Autodesk Inventor part; units mm, degrees
ref_plane "YZ Plane" through (0, 0, 0) normal (1, 0, 0) x (0, 1, 0)
ref_plane "XZ Plane" through (0, 0, 0) normal (0, 1, 0) x (-1, 0, 0)
ref_plane "XY Plane" through (0, 0, 0) normal (0, 0, 1) x (1, 0, 0)
sketch "Sketch1" plane through (0, 0, 0) normal (0, 1, 0) x (-1, 0, 0)
  line L0 (0, 0) -> (15.5956, 0)
  line L1 (15.5956, 0) -> (15.5956, -46.7868)
  line L2 (15.5956, -46.7868) -> (0, -46.7868)
  line L3 (0, -46.7868) -> (0, 0)
  dimension "d0" = 15.5956
  dimension "d7" = 46.7868
extrude "Extrusion1" add sketch "Sketch1" along normal blind 3.236
sketch "Sketch2" plane through (0, 3.236, 0) normal (0, 1, 0) x (1, 0, 0)
  line L0 (-15.5956, 0) -> (0, 0) construction
  line L1 (-15.5956, 0) -> (-11.6967, 0) construction
  line L2 (-11.6967, 0) -> (-11.6967, 3.8989) construction
  line L3 (-11.6967, 3.8989) -> (-15.5956, 3.8989) construction
  line L4 (-15.5956, 3.8989) -> (-15.5956, 0) construction
  circle A0 centre (-11.6967, 3.8989) radius 2.4498
  dimension "d10" = 3.8989
  dimension "d11" = 3.8989
  dimension "d12" = 4.8997
extrude "Extrusion2" add sketch "Sketch2" along normal blind 1.9837
pattern_linear "Rectangular Pattern1" count 6 spacing 7.7978 along (0, 0, -1) count 2 spacing 7.7978 along (1, 0, 0) of "Extrusion2"
shell "Shell1" thickness 1.4732 removed faces 1 at (-5.1985, 0, -31.1912)
sketch "Sketch3" plane through (-14.1224, 1.7628, -1.4732) normal (0, -1, 0) x (1, 0, 0)
  circle A0 centre (10.2235, -2.4257) radius 2.4498 construction
  circle A1 centre (2.4257, -10.2235) radius 2.4498 construction
  line L0 (10.2235, -2.4257) -> (2.4257, -10.2235) construction
  circle A2 centre (6.3246, -6.3246) radius 3.064
  circle A3 centre (6.3246, -6.3246) radius 2.4498
  point P0 (14.1224, 1.4732)
  dimension "d22" = 4.8997
extrude "Extrusion3" add sketch "Sketch3" along normal up to surface (1.7628 mm away)
pattern_linear "Rectangular Pattern2" count 5 spacing 7.7978 along (0, 0, -1) of "Extrusion3"
equation "\"d0\" = 2 * d1"
equation "\"d7\" = 6 * d1"
equation "\"d8\" = d2"
equation "\"d10\" = 0.5 * d1"
equation "\"d11\" = 0.5 * d1"
equation "\"d12\" = d3"
equation "\"d13\" = d4"
equation "\"d17\" = d1"
equation "\"d20\" = d1"
equation "\"d21\" = d5"
equation "\"d22\" = d3"
equation "\"d23\" = d4"
equation "\"d27\" = d1"
equation "\"d1\" = 7.7978"
equation "\"d2\" = 3.23596"
equation "\"d3\" = 4.89966"
equation "\"d4\" = 1.98374"
equation "\"d5\" = 1.4732"
equation "\"d6\" = 1.23952"
properties part number "2x6 short white pegged" material "ABS Plastic"
CAD build for the part. Positions are in the model's coordinates, mm. A direction names the side the tool comes from. Give positions to 0.01 mm unless a question says otherwise; leave off trailing zeros. Use a Markdown table: item, result.
1. Wall check: L1, parallel to X at y = 2.3, z = -19.5; L2, parallel to X at y = 1, z = -10.5; L3, parallel to Z at x = -3.75, y = 4.5. Give the ranges that are in metal, low to high. Write a range as [from, to].
Check result:
| item | result |
|---|---|
| L1 | x = [-15.6, -12.67], [-10.72, -4.88], [-2.92, 0] |
| L2 | x = [-15.6, -14.12], [-9.24, -6.35], [-1.47, 0] |
| L3 | z = [-45.33, -40.44], [-37.54, -32.64], [-29.74, -24.85], [-21.94, -17.05], [-14.14, -9.25], [-6.34, -1.45] |
2. Slice it at A-A (y = 1.1). Give the number of separate pieces and of enclosed holes in the cut face, plus the area to 3 significant figures.
Check result:
| item | result |
|---|---|
| separate pieces | 6 |
| enclosed holes | 6 |
| area | 228 mm^2 |
3. Which spindle directions (+Z, -Z, +X, -X, +Y, -Y) get a long thin tool onto all of the face, cutting with end or side? Do faces 1 (the flat face through (-8, 3.236, -23)), 2 (the flat face through (-12, 5.22, -43)), 3 (the cylindrical face through (-4.03, 2.74, -10.73)). Say none if no direction does.
Check result:
| item | result |
|---|---|
| face 1 | +Y |
| face 2 | +Z, -Z, +X, -X, +Y |
| face 3 | -Y |
4. Mould opens along Z. For faces 4 (the flat face through (-8, 1.763, -39)), 5 (the flat face through (0, 2, -24)) say: pulls with the +Z half, pulls with the -Z half, needs draft (parallel to the pull), parting line crosses it, or undercut.
Check result:
| item | result |
|---|---|
| face 4 | undercut |
| face 5 | needs draft |
5. Flat gauge pins, fed straight in: pin 1 (1.6 mm diameter, centred on x = -4, z = -4.5, fed in from -Y); pin 2 (0.6 mm diameter, centred on x = -4, z = -35.5, fed in from -Y); pin 3 (0.5 mm diameter, centred on x = -5, y = 1, fed in from +Z). Where does each tip first touch, or does it go through?
Check result:
| item | result |
|---|---|
| pin 1 | stops at y = 1.76 |
| pin 2 | stops at y = 3.75 |
| pin 3 | stops at z = 0 |
